The listing builds one solid part. Answer for the finished solid, in the listing's coordinates (mm). Face numbers are marked on the shaded views. Coordinates: 2 decimals unless noted, no trailing zeros. Order: outer loops, then holes, each group sorted by start corner. A loop starts at its lowest first (then second) coordinate and runs counter-clockwise, first axis right, second up.
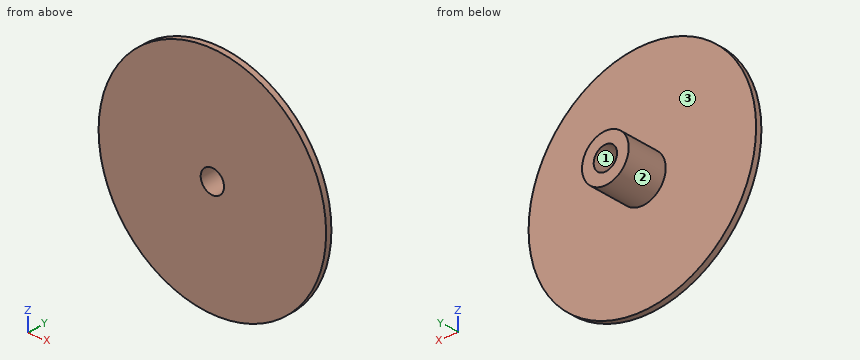
from build123d import *

# Parameters (mm, degrees)
F0_R     = 123.825
F1_DEPTH = 3.175
F2_R     = 25.4
F3_DEPTH = 50.8
F4_R     = 12.7
F5_DEPTH = 63.5


with BuildPart() as f1:
    # F0 (on Front) → F1 (new body, symmetric)
    with BuildSketch(Plane.XZ):
        Circle(F0_R)
    extrude(amount=F1_DEPTH, both=True)

    # F2 (on face) → F3 (join)
    with BuildSketch(Plane.XZ.offset(3.175)):
        Circle(F2_R)
    extrude(amount=-F3_DEPTH)

    # F4 (on face) → F5 (cut, symmetric)
    with BuildSketch(Plane.XZ.offset(3.175)):
        Circle(F4_R)
    extrude(amount=F5_DEPTH, both=True, mode=Mode.SUBTRACT)


solid = f1.part
(1) Find section C-C on y = 42. Determine the outline of the cut face in (x, z), then the cut area to 3 significant figures.
(2) Find section D-D on z = 101. Determine the outline of the cut face in (x, y) (3 decimals), then the cut area to 3 significant figures.
(3) Given pin 1 Ø12 at (x, y) = (-34.5, 26) entering from +Z; pin 2 Ø6 at (x, y) = (-15.5, 36) entering from +Z; pin 3 Ø8 at (x, z) = (-82, 84) entering from +Y (3 decimals); pin 4 Ø1 at (y, z) = (29, -21.5) entering from +X, each flat-ended and moving along its own axis, determine where each tip first touches the part or whether it passes through.
(4) Find section B-B on x = 0. Determine the outline of the cut face in (y, z) (3 decimals), then the cut area to 3 significant figures.
(5) The mould has two halves that part along X. Classify the marked faces 1, 2 and 3: pulls with the +X half, pulls with the -X half, needs draft (parallel to the pull), parting line crosses it, or undercut.
(6) Find section A-A on z = 0. Determine the outline of the cut face in (x, y) (3 decimals).
(7) Find the intervals of material crossed by probe 1 along Y at (x, z) = (97, 16) (3 decimals); probe 2 along Z at (x, y) = (0, 29); probe 3 along X at (y, z) = (28.5, 7), in increasing order.
Resolved:
1. outline: circle Ø50.8 at (0, 0); hole circle Ø25.4 at (0, 0)
1. area: 1,520 mm2
2. outline: (-71.635, -3.175) - (71.635, -3.175) - (71.635, 3.175) - (-71.635, 3.175) - close
2. area: 910 mm2
3. pin 1: passes through
3. pin 2: stops at z = 22.11
3. pin 3: stops at y = 3.175
3. pin 4: stops at x = 14.29
4. outline: (-3.175, -123.825) - (3.175, -123.825) - (3.175, -25.4) - (47.625, -25.4) - (47.625, -12.7) - (-3.175, -12.7) - close; (-3.175, 12.7) - (47.625, 12.7) - (47.625, 25.4) - (3.175, 25.4) - (3.175, 123.825) - (-3.175, 123.825) - close
4. area: 2,540 mm2
5. face 1: undercut
5. face 2: parting line crosses it
5. face 3: needs draft
6. outline: (-123.825, -3.175) - (-12.7, -3.175) - (-12.7, 47.625) - (-25.4, 47.625) - (-25.4, 3.175) - (-123.825, 3.175) - close; (12.7, -3.175) - (123.825, -3.175) - (123.825, 3.175) - (25.4, 3.175) - (25.4, 47.625) - (12.7, 47.625) - close
7. probe 1: y = -3.175 to 3.175
7. probe 2: z = -25.4 to -12.7, 12.7 to 25.4
7. probe 3: x = -24.42 to -10.6, 10.6 to 24.42
